Could you check a few things on this model? Use its own coordinates, in mm. Face numbers are marked on the shaded views. Coordinates: 2 decimals unless noted, no trailing zeros. Write each loop counter-clockwise with the first axis right and the second up, starting at its lowest first coordinate (ties: lowest second). Pieces come first, ordered by that corner, then holes. Notation, with made-up numbers: (-32.5, 41) - (-8.5, 41) arc R5 cw to (-8.5, 48) - close; hole circle Ø3 at (-9, -18). An arc over 180 degrees is marked (long way). Write item = value, one per line. Start each with the question number.
```python
from build123d import *

# Parameters (mm, degrees)
F0_W          = 93.5181863606
F0_H          = 99.5218157768
F1_DEPTH      = 127
F2_R          = 24.7334517627
F3_DEPTH      = 186.5019382
F3_DEPTH_BACK = 41.98141


# Not quite as in the source:
# - an extrude ends at something that could not be found from the text; its depth is read off the source's solid


with BuildPart() as f1:
    # F0 (on Top) → F1 (new body)
    with BuildSketch(Plane.XY):
        with Locations((3.8100015372, -1.3854540884)):
            Rectangle(F0_W, F0_H)
    extrude(amount=F1_DEPTH)

    # F2 (on face) → F3 (join, two sides)
    with BuildSketch(Plane.YZ.offset(50.5690947175)) as f3_sk:
        with Locations((-24.546951997, 83.1744330844)):
            Circle(F2_R)
    extrude(amount=F3_DEPTH)
    extrude(f3_sk.sketch, amount=-F3_DEPTH_BACK)


solid = f1.part
```
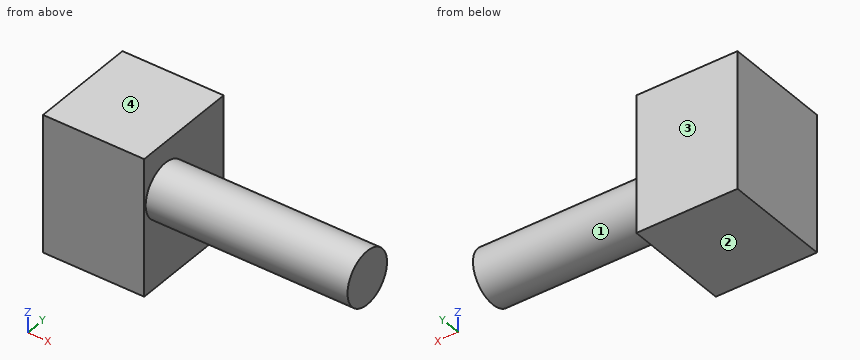
1) If I drill on probe 1 along Z at (x, y) = (119, -26); probe 2 along X at (y, z) = (-39, 121); probe 3 along Y at (x, z) = (117, 72), over which ranges is the centre line in solid material (lowest first)? Write a range as [from, to].
2) Suppose I cut it at A-A on y = -20. Please give me the cut outline in (x, z).
3) Thinking about a two-plate mould opening in Z: for the marked faces 1, 2, 3 and 4, which applies, +Z half, -Z half, draft (parallel to the pull), parting line (faces both ways), or undercut?
4) Suppose I cut it at D-D on x = 124. Please give me the cut outline in (y, z).
5) For P1, Ø12, axis at x = 175, y = 1.5, coming from the -Z side; P2, Ø8, axis at x = 177.5, z = 52.5, coming from the +Y side, each with a flat end and sliding along its axis, tell me the tip position at first contact or that it passes through.
6) Suppose I cut it at B-B on z = 102. Please give me the cut outline in (x, y), plus the area to 3 significant figures.
7) Suppose I cut it at C-C on y = 15. Please give me the cut outline in (x, z).
Reply:
q1.probe_1 = [58.48, 107.87]
q1.probe_2 = [-42.95, 50.57]
q1.probe_3 = [-46.61, -2.48]
q2.outline = (-42.95, 0) - (50.57, 0) - (50.57, 58.86) - (237.07, 58.86) - (237.07, 107.49) - (50.57, 107.49) - (50.57, 127) - (-42.95, 127) - close
q3.face_1 = parting line
q3.face_2 = -Z half
q3.face_3 = draft
q3.face_4 = +Z half
q4.outline = circle Ø49.47 at (-24.55, 83.17)
q5.P1 = 68.69
q5.P2 = through
q6.outline = (-42.95, -51.15) - (50.57, -51.15) - (50.57, -40.59) - (237.07, -40.59) - (237.07, -8.51) - (50.57, -8.51) - (50.57, 48.38) - (-42.95, 48.38) - close
q6.area = 15,300 mm^2
q7.outline = (-42.95, 0) - (50.57, 0) - (50.57, 127) - (-42.95, 127) - close
